Verification items for this drawing (mm, ordinates from the low corner). A direction names the side the tool comes from. Give positions to 0.01 mm unless a question says otherwise; leave off trailing zeros. Write each loop counter-clockwise with the first axis right and the second up, starting at its lowest first coordinate (ties: lowest second). Pieces come first, ordered by that corner, then holes. Notation, with made-up numbers: (-1.5, 64.25) -> (16.5, 64.25) arc R21 cw to (16.5, 97.25) -> close; hole circle Ø8 at (-8.5, -27.5). An arc over 180 degrees is marked (long way). Write item = value, one per line.
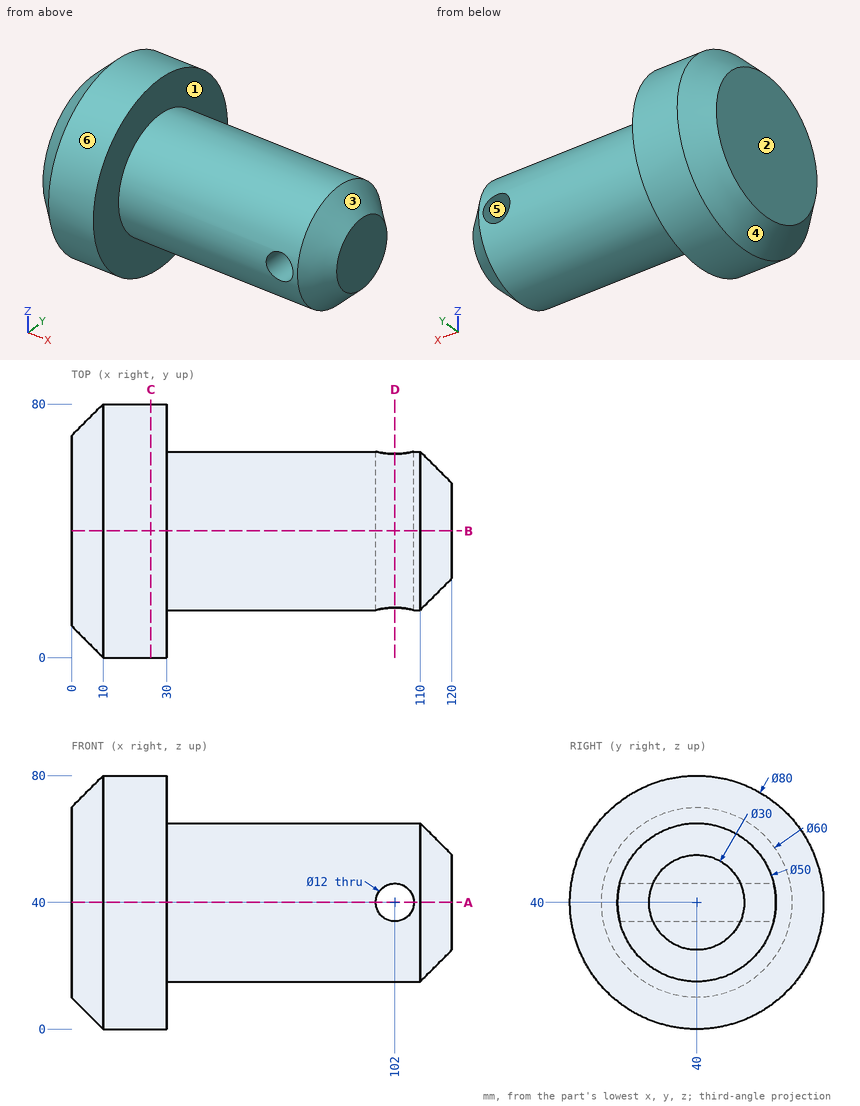
Item 1: Mould release check, pull along X, two halves, no side actions. Record for the marked faces 3, 4, 5 and 6: +X half, -X half, draft (parallel to the pull), parting line (faces both ways), or undercut.
Response values:
face_3 = +X half
face_4 = -X half
face_5 = undercut
face_6 = draft
Item 2: Set-up check for the marked faces 1 and 2: record each of +Z, -Z, +X, -X, +Y, -Y from which the full face is reachable in a straight line by a thin tool's end or side.
Response values:
face_1 = +X
face_2 = +Z, -Z, -X, +Y, -Y
Item 3: Sectioned sample at A-A on z = 40. Record the cut outline in (x, y), then the cut area to 3 significant figures.
Response values:
outline = (0, 10) -> (10, 0) -> (30, 0) -> (30, 15) -> (96, 15) -> (96, 65) -> (30, 65) -> (30, 80) -> (10, 80) -> (0, 70) -> close; (108, 15) -> (110, 15) -> (120, 25) -> (120, 55) -> (110, 65) -> (108, 65) -> close
area = 6,100 mm^2
Item 4: Go/stop test with flat-tipped pins: P1, Ø8, axis at x = 70, z = 17.5, coming from the +Y side; P2, Ø4, axis at x = 16.5, z = 60, coming from the -Y side; P3, Ø1, axis at x = 56.5, z = 61.5, coming from the -Y side; P4, Ø1.5, axis at y = 45.5, z = 49.5, coming from the -X side. Record where each tip stops, or that it passes through.
Response values:
P1 = 56.82
P2 = 4.28
P3 = 26.44
P4 = 0
Item 5: Sectioned sample at D-D on x = 102. Record the cut outline in (y, z), then the cut area to 3 significant figures.
Response values:
outline = (15.73, 34) arc R25 ccw to (64.27, 34) -> close; (15.73, 46) -> (64.27, 46) arc R25 ccw to start
area = 1,370 mm^2
Item 6: Sectioned sample at C-C on x = 25. Record the cut outline in (y, z), then the cut area to 3 significant figures.
Response values:
outline = circle Ø80 at (40, 40)
area = 5,030 mm^2
Item 7: Sectioned sample at B-B on y = 40. Record the cut outline in (x, z).
Response values:
outline = (0, 10) -> (10, 0) -> (30, 0) -> (30, 15) -> (110, 15) -> (120, 25) -> (120, 55) -> (110, 65) -> (30, 65) -> (30, 80) -> (10, 80) -> (0, 70) -> close; hole circle Ø12 at (102, 40)
Item 8: Material ranges on line 1 (X direction, y = 43.5, z = 40); line 2 (Z direction, x = 102.5, y = 59.5); line 3 (Z direction, x = 102, y = 47), recorded low to high.
Response values:
line_1 = 0 to 96, 108 to 120
line_2 = 24.36 to 34.02, 45.98 to 55.64
line_3 = 16 to 34, 46 to 64
